from build123d import *

# Parameters (mm, degrees)
FILLET1_R    = 0.2
SKETCH3_W    = 1.03
SKETCH3_H    = 4.3
SKETCH4_W    = 1.03
SKETCH4_H    = 1.966638154
RECPAT_COUNT = 2
RECPAT_ANGLE = 90


with BuildPart() as part:
    # BodySke → Base-Revolve (revolve)
    with BuildSketch(Plane.XY):
        with BuildLine():
            Line((3.1, 2), (3.1, 4))
            Line((3.1, 4), (1.555305874, 4))
            ThreePointArc((1.555305874, 4), (1.392873227, 3.961271902), (1.265388955, 3.853420195))
            ThreePointArc((1.265388955, 3.853420195), (0.324444487, 2.027933456), (0, 0))
            Line((0, 0), (53.1, 0))
            Line((53.1, 0), (53.1, 2))
            Line((53.1, 2), (3.1, 2))
        make_face()
    revolve(axis=Axis((-25.4, 0, 0), (1, 0, 0)))

    # Fillet1
    fillet1_edges = [part.edges().sort_by_distance(p)[0] for p in [
        (3.1, -2, 0),
    ]]
    fillet(fillet1_edges, radius=FILLET1_R)

    # Sketch3 → Recess section 0
    with BuildSketch(Plane(origin=(0, 0, 0), x_dir=(0, 0, -1), z_dir=(1, 0, 0))):
        Rectangle(SKETCH3_W, SKETCH3_H)
    # Sketch4 → Recess section 1
    with BuildSketch(Plane(origin=(2.34, 0, 0), x_dir=(0, 0, -1), z_dir=(1, 0, 0))):
        Rectangle(SKETCH4_W, SKETCH4_H)
    recess = loft(mode=Mode.SUBTRACT)

    # RecPat: Recess ×2 about axis
    recpat_axis = Axis((0, 0, 0), (1, 0, 0))
    for i in range(1, RECPAT_COUNT):
        add(recess.rotate(recpat_axis, i * RECPAT_ANGLE / (RECPAT_COUNT - 1)), mode=Mode.SUBTRACT)

    # RecCorSke → RecessCore (revolve, cut)
    with BuildSketch(Plane.XY):
        Polygon((0, 0), (0, 1.01462874), (2.34, 0.851), (2.616506661, 0), align=None)
    revolve(axis=Axis((-3.175, 0, 0), (1, 0, 0)), mode=Mode.SUBTRACT)


solid = part.part
The model under review builds one solid part; all positions refer to its coordinate system, in mm. A direction names the side the tool comes from. Coordinates: 2 decimals unless noted, no trailing zeros. Write each loop counter-clockwise with the first axis right and the second up, starting at its lowest first coordinate (ties: lowest second). Pieces come first, ordered by that corner, then holes. Notation, with made-up numbers: (57.5, 1.25) -> (64.5, 1.25) arc R4 ccw to (64.5, 8.25) -> close; hole circle Ø10 at (-30, -7). An arc over 180 degrees is marked (long way). Answer in a Markdown table with one row per item.
1. We need section A-A, the plane x = 4.5. State the section outline as (y, z) points, and give its area (3 significant figures).
Answers below:
| item | result |
|---|---|
| outline | circle Ø4 at (0, 0) |
| area | 12.6 mm^2 |
2. Clearance check with flat-ended pins moving along their axes: pin 1 Ø1.5 at (x, z) = (33, 3) entering from +Y; pin 2 Ø2 at (x, z) = (30.5, -2) entering from -Y; pin 3 Ø1.5 at (y, z) = (-0.5, -3) entering from -X; pin 4 Ø1.5 at (x, z) = (28.5, 1.5) entering from -Y. State where each tip first meets the part, or that it passes through.
Answers below:
| item | result |
|---|---|
| pin 1 | passes through |
| pin 2 | stops at y = -1.73 |
| pin 3 | stops at x = 0.42 |
| pin 4 | stops at y = -1.85 |
3. Draft analysis for pull direction Y (two halves, no side actions). For faces 3 (the cylindrical face through (2.317, -0.867, -3.905)), 4 (the flat face through (1.3, 0, -1.5)), 5 (the flat face through (53.1, 0, 0)), state which applies: +Y half, -Y half, draft (parallel to the pull), parting line (faces both ways), or undercut.
Answers below:
| item | result |
|---|---|
| face 3 | parting line |
| face 4 | undercut |
| face 5 | draft |
4. For faces 1 (the flat face through (3.1, -2, -2)), 2 (the flat face through (1.3, 1.5, 0)), list the 3-axis set-ups (+Z, -Z, +X, -X, +Y, -Y) from which the entire face can be reached by the end or side of a thin tool; tool diameter is ignored.
Answers below:
| item | result |
|---|---|
| face 1 | +X |
| face 2 | -X |
5. Wall thickness on probe 1 along Z at (x, y) = (48, 0.25); probe 2 along X at (y, z) = (1.75, 2.75); probe 3 along X at (y, z) = (-3.5, 0.5): over which ranges is each line inside the solid? List them lowest first. Write a range as [from, to].
Answers below:
| item | result |
|---|---|
| probe 1 | z = [-1.98, 1.98] |
| probe 2 | x = [0.88, 3.1] |
| probe 3 | x = [1.05, 3.1] |
